Check sheet for the drawn part. Datum: minimum x, y, z corner. Units: mm. A direction names the side the tool comes from. Coordinates: 2 decimals unless noted, no trailing zeros. Loops run counter-clockwise (first coordinate to the right, second up) from the corner with the lowest first, then second, coordinate; pieces in that order, holes last. Notation, with made-up numbers: (78, -29.5) -> (136, -29.5) arc R12 cw to (136, -23.5) -> close; hole circle Ø4 at (-2.5, 12). An arc over 180 degrees is marked (long way). Use CSV: the item, a comma, the result in double quotes. Start each with the question number.
1. Sectioned sample at D-D, the plane y = 20. Record the cut outline in (x, z).
2. Sectioned sample at A-A, the plane z = 9. Record the cut outline in (x, y).
3. Gauge pin test, flat ends, axial feed: pin 1 (6 mm diameter, centred on x = 19, y = 30.5, fed in from +Z); pin 2 (14 mm diameter, centred on x = 12, y = 24, fed in from +Z); pin 3 (6 mm diameter, centred on x = 21.5, z = 19, fed in from +Y). Record the tip position at first contact, or that the pin passes through.
4. Sectioned sample at C-C, the plane z = 5.5. Record the cut outline in (x, y), and give its area (3 significant figures).
5. Release check for a two-part mould opening along Y. For the marked faces 1, 2 and 3 record: pulls with the +Y half, pulls with the -Y half, needs draft (parallel to the pull), parting line crosses it, or undercut.
6. Thickness scan on L1, parallel to Y at x = 22.75, z = 18.5; L2, parallel to Z at x = 5.75, y = 23.5; L3, parallel to Z at x = 18, y = 7.5. Record the ranges inside material, lowest first.
7. Set-up check for the marked faces 4, 5 and 6: record each of +Z, -Z, +X, -X, +Y, -Y from which the full face is reachable in a straight line by a thin tool's end or side.
8. Sectioned sample at B-B, the plane x = 23. Record the cut outline in (y, z), and give its area (3 significant figures).
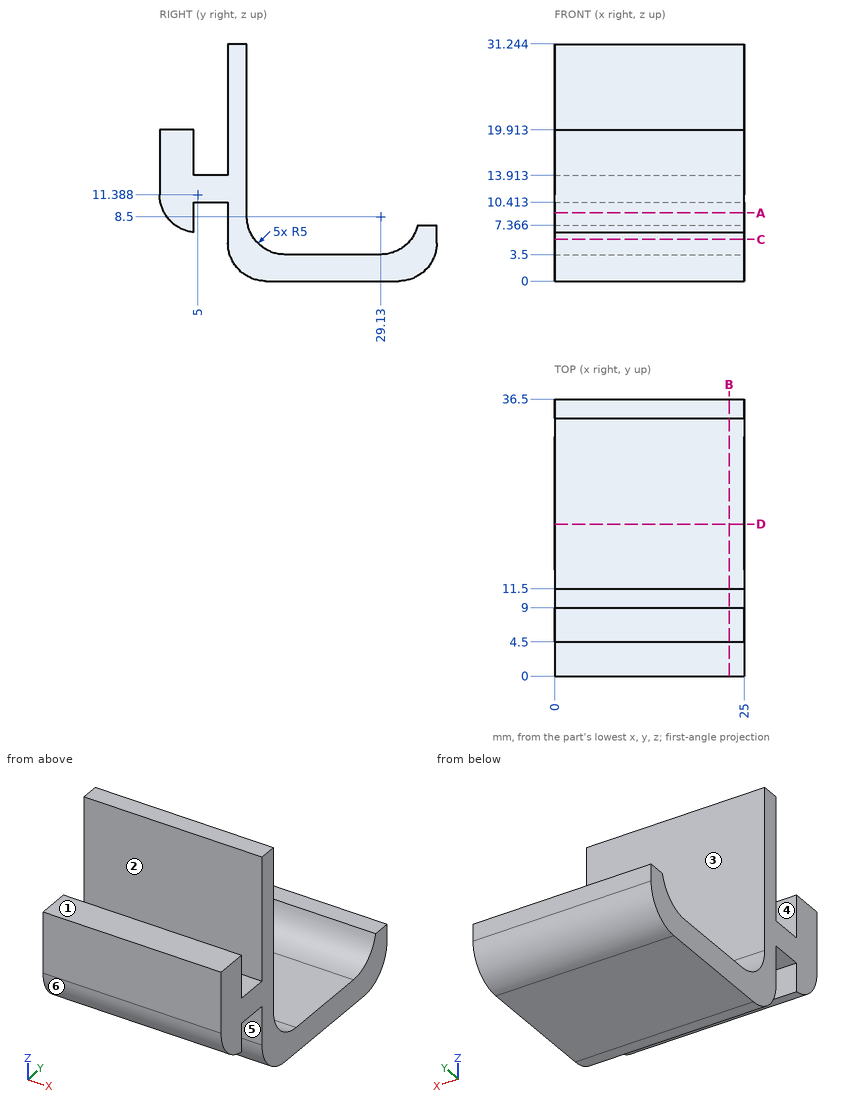
Completed:
1,outline,"(0, 0) -> (25, 0) -> (25, 3.5) -> (0, 3.5) -> close"
2,outline,"(0, 0.61) -> (25, 0.61) -> (25, 4.5) -> (0, 4.5) -> close; (0, 9) -> (25, 9) -> (25, 11.5) -> (0, 11.5) -> close"
3,pin 1,"z = 6.07"
3,pin 2,"z = 3.86"
3,pin 3,"y = 11.5"
4,outline,"(0, 9) -> (25, 9) -> (25, 12.5) -> (0, 12.5) -> close; (0, 33.13) -> (25, 33.13) -> (25, 36.5) -> (0, 36.5) -> close"
4,area,"172 mm²"
5,face 1,"needs draft"
5,face 2,"undercut"
5,face 3,"pulls with the +Y half"
6,L1,"0 to 4.5, 9 to 11.5"
6,L2,"0 to 3.5"
6,L3,"10.41 to 13.91"
7,face 4,"+Z, +X, -X"
7,face 5,"-Z, +X, -X"
7,face 6,"-Z, +X, -X, -Y"
8,outline,"(0, 11.39) arc R5 ccw to (4.5, 6.41) -> (4.5, 10.41) -> (9, 10.41) -> (9, 5) arc R5 ccw to (14, 0) -> (31.5, 0) arc R5 ccw to (36.5, 5) -> (36.5, 7.37) -> (34, 7.37) arc R5 cw to (29.13, 3.5) -> (16.5, 3.5) arc R5 cw to (11.5, 8.5) -> (11.5, 31.24) -> (9, 31.24) -> (9, 13.91) -> (4.5, 13.91) -> (4.5, 19.91) -> (0, 19.91) -> close"
8,area,"246 mm²"
